Study the drawing (mm; zero at the part's minimum x, y, z) and answer. A direction names the side the tool comes from. Round coordinates to 2 decimals unless told otherwise and drop trailing zeros. Write each loop counter-clockwise with the first axis right and the second up, starting at its lowest first coordinate (ties: lowest second). Pieces come first, ordered by that corner, then holes. Notation, with made-up numbers: (-21, 81.5) - (7, 81.5) arc R9 ccw to (7, 98.5) - close; hole circle Ø1 at (-28, 54.25). An arc over 180 degrees is marked (long way). Return JSON: item names as keys, results as strings. Group by question number.
(1) Section A-A, the plane y = 36 is taken. Write down the section's boundary in (x, z), then the cut area to 3 significant figures.
(2) Section C-C, the plane x = 33 is taken. Write down the section's boundary in (y, z) (3 decimals), then the cut area to 3 significant figures.
(3) Find the intervals of material crossed by line 1 along Y through (x, z) = (8.5, 18.5); line 2 along X through (y, z) = (2, 16); line 3 along Y through (x, z) = (44, 36.5), in increasing order. Write a range as [from, to].
(4) Each of these flat-tipped pins is pushed along its axis until it touches: pin 1 (5 mm diameter, centred on x = 48, z = 22.5, fed in from -Y); pin 2 (5 mm diameter, centred on x = 6, y = 34, fed in from +Z); pin 3 (1 mm diameter, centred on y = 32, z = 26, fed in from +X). Where does it stop, or does it pass through?
(5) Which of the six approach directions +Z, -Z, +X, -X, +Y, -Y give full straight-line access (tool end or side, diameter ignored) to the marked faces 5, 6 and 7?
(6) Determine the mould class of the marked faces 1, 2, 3 and 4 for opening direction Y: +Y half, -Y half, draft (parallel to the pull), parting line (faces both ways), or undercut.
(7) Section B-B, the plane z = 13 is taken. Write down the section's boundary in (x, y).
(8) Section D-D, the plane x = 8 is taken. Write down the section's boundary in (y, z), then the cut area to 3 significant figures.
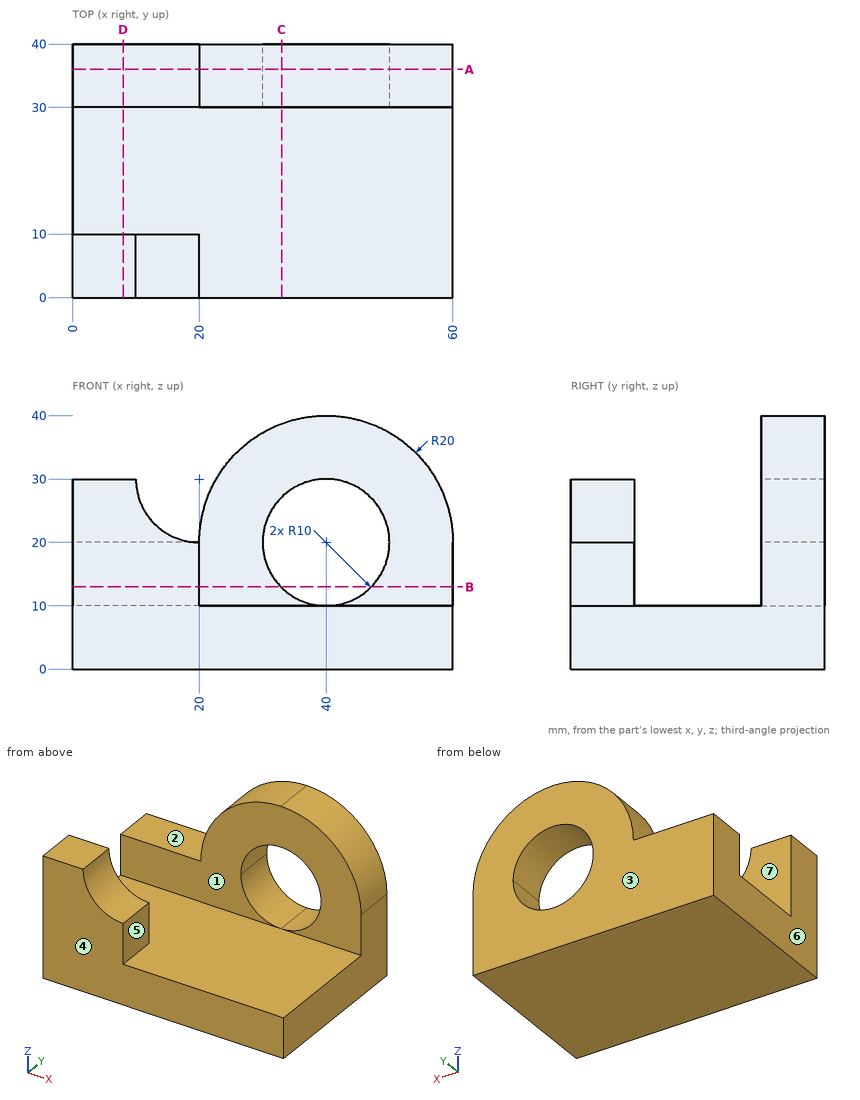
Working result:
{
 "1": {"outline": "(0, 0) - (60, 0) - (60, 20) arc R20 ccw to (20, 20) - (0, 20) - close; hole circle Ø20 at (40, 20)", "area": "1,510 mm^2"},
 "2": {"outline": "(0, 0) - (40, 0) - (40, 12.859) - (30, 12.859) - (30, 10) - (0, 10) - close; (30, 27.141) - (40, 27.141) - (40, 38.735) - (30, 38.735) - close", "area": "545 mm^2"},
 "3": {"line 1": "y = [0, 10], [30, 40]", "line 2": "x = [0, 20]", "line 3": "y = [30, 40]"},
 "4": {"pin 1": "stops at y = 30", "pin 2": "stops at z = 20", "pin 3": "stops at x = 59.23"},
 "5": {"face 5": "+Z, +X, -Y", "face 6": "+Z, -Z, -X, +Y, -Y", "face 7": "+Z, +X, -X"},
 "6": {"face 1": "undercut", "face 2": "draft", "face 3": "+Y half", "face 4": "-Y half"},
 "7": {"outline": "(0, 0) - (20, 0) - (20, 10) - (0, 10) - close; (0, 30) - (32.86, 30) - (32.86, 40) - (0, 40) - close; (47.14, 30) - (60, 30) - (60, 40) - (47.14, 40) - close"},
 "8": {"outline": "(0, 0) - (40, 0) - (40, 20) - (30, 20) - (30, 10) - (10, 10) - (10, 30) - (0, 30) - close", "area": "700 mm^2"}
}
